```python
from build123d import *

# Parameters (mm, degrees)
SKIZZE1_W                       = 250
SKIZZE1_H                       = 150
AUFSATZ_LINEAR_AUSTRAGEN1_DEPTH = 12


with BuildPart() as part:
    # Skizze1 → Aufsatz-Linear austragen1 (new body)
    with BuildSketch(Plane(origin=(0, 0, 0), x_dir=(1, 0, 0), z_dir=(0, 1, 0))):
        Rectangle(SKIZZE1_W, SKIZZE1_H)
        with BuildLine():
            Line((27.95, 10.5), (27.95, 20.5))
            ThreePointArc((27.95, 20.5), (29.5, 22.05), (31.05, 20.5))
            Line((31.05, 20.5), (31.05, 10.5))
            ThreePointArc((31.05, 10.5), (29.5, 8.95), (27.95, 10.5))
        make_face(mode=Mode.SUBTRACT)
        with BuildLine():
            Line((62.05, 20.5), (62.05, 10.5))
            ThreePointArc((62.05, 10.5), (60.5, 8.95), (58.95, 10.5))
            Line((58.95, 10.5), (58.95, 20.5))
            ThreePointArc((58.95, 20.5), (60.5, 22.05), (62.05, 20.5))
        make_face(mode=Mode.SUBTRACT)
        with BuildLine():
            Line((58.95, -20.5), (58.95, -10.5))
            ThreePointArc((58.95, -10.5), (60.5, -8.95), (62.05, -10.5))
            Line((62.05, -10.5), (62.05, -20.5))
            ThreePointArc((62.05, -20.5), (60.5, -22.05), (58.95, -20.5))
        make_face(mode=Mode.SUBTRACT)
        with BuildLine():
            Line((27.95, -20.5), (27.95, -10.5))
            ThreePointArc((27.95, -10.5), (29.5, -8.95), (31.05, -10.5))
            Line((31.05, -10.5), (31.05, -20.5))
            ThreePointArc((31.05, -20.5), (29.5, -22.05), (27.95, -20.5))
        make_face(mode=Mode.SUBTRACT)
        with BuildLine():
            Line((56, 5), (56, -5))
            ThreePointArc((56, -5), (45, -16), (34, -5))
            Line((34, -5), (34, 5))
            ThreePointArc((34, 5), (45, 16), (56, 5))
        make_face(mode=Mode.SUBTRACT)
    extrude(amount=AUFSATZ_LINEAR_AUSTRAGEN1_DEPTH)


solid = part.part
```
Input: part model. Units: mm. Frame: model coordinates. A direction names the side the tool comes from. Coordinates: 2 decimals unless noted, no trailing zeros. Write each loop counter-clockwise with the first axis right and the second up, starting at its lowest first coordinate (ties: lowest second). Pieces come first, ordered by that corner, then holes. Notation, with made-up numbers: (77.5, 25.5) -> (132.5, 25.5) arc R21 ccw to (132.5, 47.5) -> close; hole circle Ø4 at (-7, 79). An arc over 180 degrees is marked (long way). Answer as a JSON object with one key per item and string values.
1. Mould query, pull axis X, two halves, no side actions, for faces 3 (the face through (31.05, 6, 15)), 4 (the face through (125, 6, 1)), 5 (the face through (-2, 0, -1)). Classes: released by +X, released by -X, zero draft, split by the parting line, or undercut.
Result set:
{"face 3": "undercut", "face 4": "released by +X", "face 5": "zero draft"}
2. Section A-A on y = 8.25. Return the cut outline in (x, z).
Result set:
{"outline": "(-125, -75) -> (125, -75) -> (125, 75) -> (-125, 75) -> close; hole (27.95, -20.5) arc R1.55 ccw to (31.05, -20.5) -> (31.05, -10.5) arc R1.55 ccw to (27.95, -10.5) -> close; hole (27.95, 10.5) arc R1.55 ccw to (31.05, 10.5) -> (31.05, 20.5) arc R1.55 ccw to (27.95, 20.5) -> close; hole (34, -5) arc R11 ccw to (56, -5) -> (56, 5) arc R11 ccw to (34, 5) -> close; hole (58.95, -20.5) arc R1.55 ccw to (62.05, -20.5) -> (62.05, -10.5) arc R1.55 ccw to (58.95, -10.5) -> close; hole (58.95, 10.5) arc R1.55 ccw to (62.05, 10.5) -> (62.05, 20.5) arc R1.55 ccw to (58.95, 20.5) -> close"}
3. Section B-B on x = 45. Return the cut outline in (y, z).
Result set:
{"outline": "(0, -75) -> (12, -75) -> (12, -16) -> (0, -16) -> close; (0, 16) -> (12, 16) -> (12, 75) -> (0, 75) -> close"}
4. Material intervals for line 1 (X direction, y = 7.5, z = -2.5); line 2 (X direction, y = 11, z = -17); line 3 (X direction, y = 10, z = 12), sorted ascending. Write a range as from..to.
Result set:
{"line 1": "x = -125..34, 56..125", "line 2": "x = -125..27.95, 31.05..58.95, 62.05..125", "line 3": "x = -125..27.95, 31.05..36.51, 53.49..58.95, 62.05..125"}
5. Access query for faces 1 (the face through (56, 6, 0)), 2 (the face through (-125, 6, 1)). Directions: +Z, -Z, +X, -X, +Y, -Y. A direction counts if a zero-diameter tool reaches every point of the face in a straight line with its end or side. Return the directions, or none.
Result set:
{"face 1": "+Y, -Y", "face 2": "+Z, -Z, -X, +Y, -Y"}
